```python
from build123d import *

# Parameters (mm, degrees)
SKETCH1_R           = 4
SKETCH1_R_2         = 2
BOSS_EXTRUDE1_DEPTH = 3.175


with BuildPart() as part:
    # Sketch1 → Boss-Extrude1 (new body)
    with BuildSketch(Plane.XY):
        with BuildLine():
            Line((144, -229.5), (144, -248.5))
            ThreePointArc((144, -248.5), (146.196699141, -253.803300859), (151.5, -256))
            Line((151.5, -256), (200.5, -256))
            ThreePointArc((200.5, -256), (205.803300859, -253.803300859), (208, -248.5))
            Line((208, -248.5), (208, -201.169519945))
            ThreePointArc((208, -201.169519945), (207.595148356, -198.73870325), (206.424301385, -196.570318591))
            Line((206.424301385, -196.570318591), (43.651971362, 13.099201355))
            ThreePointArc((43.651971362, 13.099201355), (41.025850524, 15.235874485), (37.727669977, 16))
            Line((37.727669977, 16), (-8.5, 16))
            ThreePointArc((-8.5, 16), (-13.803300859, 13.803300859), (-16, 8.5))
            Line((-16, 8.5), (-16, -8.5))
            ThreePointArc((-16, -8.5), (-13.803300859, -13.803300859), (-8.5, -16))
            Line((-8.5, -16), (0.5, -16))
            ThreePointArc((0.5, -16), (5.803300859, -18.196699141), (8, -23.5))
            Line((8, -23.5), (8, -214.5))
            ThreePointArc((8, -214.5), (10.196699141, -219.803300859), (15.5, -222))
            Line((15.5, -222), (136.5, -222))
            ThreePointArc((136.5, -222), (141.803300859, -224.196699141), (144, -229.5))
        make_face()
        Circle(SKETCH1_R, mode=Mode.SUBTRACT)
        with Locations((0, 8)):
            Circle(SKETCH1_R_2, mode=Mode.SUBTRACT)
        with Locations((160, -240)):
            Circle(SKETCH1_R, mode=Mode.SUBTRACT)
        with Locations((176, -240)):
            Circle(SKETCH1_R, mode=Mode.SUBTRACT)
        with Locations((160, -232)):
            Circle(SKETCH1_R_2, mode=Mode.SUBTRACT)
        with Locations((168, -240)):
            Circle(SKETCH1_R_2, mode=Mode.SUBTRACT)
        with Locations((160, -248)):
            Circle(SKETCH1_R_2, mode=Mode.SUBTRACT)
        with Locations((152, -240)):
            Circle(SKETCH1_R_2, mode=Mode.SUBTRACT)
        with Locations((200, -240)):
            Circle(SKETCH1_R_2, mode=Mode.SUBTRACT)
        with Locations((192, -248)):
            Circle(SKETCH1_R_2, mode=Mode.SUBTRACT)
        with Locations((192, -240)):
            Circle(SKETCH1_R, mode=Mode.SUBTRACT)
        with Locations((184, -240)):
            Circle(SKETCH1_R_2, mode=Mode.SUBTRACT)
        with Locations((192, -232)):
            Circle(SKETCH1_R_2, mode=Mode.SUBTRACT)
        with Locations((8, 0)):
            Circle(SKETCH1_R_2, mode=Mode.SUBTRACT)
        with Locations((0, -8)):
            Circle(SKETCH1_R_2, mode=Mode.SUBTRACT)
        with Locations((-8, 0)):
            Circle(SKETCH1_R_2, mode=Mode.SUBTRACT)
        with Locations((36, -212)):
            Circle(SKETCH1_R_2, mode=Mode.SUBTRACT)
        with Locations((28, -204)):
            Circle(SKETCH1_R_2, mode=Mode.SUBTRACT)
        with Locations((36, -196)):
            Circle(SKETCH1_R_2, mode=Mode.SUBTRACT)
        with Locations((44, -204)):
            Circle(SKETCH1_R_2, mode=Mode.SUBTRACT)
        with Locations((44, -188)):
            Circle(SKETCH1_R_2, mode=Mode.SUBTRACT)
        with Locations((36, -180)):
            Circle(SKETCH1_R_2, mode=Mode.SUBTRACT)
        with Locations((28, -188)):
            Circle(SKETCH1_R_2, mode=Mode.SUBTRACT)
        with Locations((44, -172)):
            Circle(SKETCH1_R_2, mode=Mode.SUBTRACT)
        with Locations((36, -164)):
            Circle(SKETCH1_R_2, mode=Mode.SUBTRACT)
        with Locations((28, -172)):
            Circle(SKETCH1_R_2, mode=Mode.SUBTRACT)
        with Locations((44, -156)):
            Circle(SKETCH1_R_2, mode=Mode.SUBTRACT)
        with Locations((36, -148)):
            Circle(SKETCH1_R_2, mode=Mode.SUBTRACT)
        with Locations((28, -156)):
            Circle(SKETCH1_R_2, mode=Mode.SUBTRACT)
        with Locations((44, -140)):
            Circle(SKETCH1_R_2, mode=Mode.SUBTRACT)
        with Locations((36, -132)):
            Circle(SKETCH1_R_2, mode=Mode.SUBTRACT)
        with Locations((28, -140)):
            Circle(SKETCH1_R_2, mode=Mode.SUBTRACT)
        with Locations((44, -124)):
            Circle(SKETCH1_R_2, mode=Mode.SUBTRACT)
        with Locations((36, -116)):
            Circle(SKETCH1_R_2, mode=Mode.SUBTRACT)
        with Locations((28, -124)):
            Circle(SKETCH1_R_2, mode=Mode.SUBTRACT)
        with Locations((44, -108)):
            Circle(SKETCH1_R_2, mode=Mode.SUBTRACT)
        with Locations((36, -100)):
            Circle(SKETCH1_R_2, mode=Mode.SUBTRACT)
        with Locations((28, -108)):
            Circle(SKETCH1_R_2, mode=Mode.SUBTRACT)
        with Locations((44, -92)):
            Circle(SKETCH1_R_2, mode=Mode.SUBTRACT)
        with Locations((36, -84)):
            Circle(SKETCH1_R_2, mode=Mode.SUBTRACT)
        with Locations((28, -92)):
            Circle(SKETCH1_R_2, mode=Mode.SUBTRACT)
        with Locations((44, -76)):
            Circle(SKETCH1_R_2, mode=Mode.SUBTRACT)
        with Locations((36, -68)):
            Circle(SKETCH1_R_2, mode=Mode.SUBTRACT)
        with Locations((28, -76)):
            Circle(SKETCH1_R_2, mode=Mode.SUBTRACT)
    extrude(amount=BOSS_EXTRUDE1_DEPTH)


solid = part.part
```
Build history of the part. All positions in model axes, mm. Round coordinates to 2 decimals unless told otherwise and drop trailing zeros. Loops run counter-clockwise (first coordinate to the right, second up) from the corner with the lowest first, then second, coordinate; pieces in that order, holes last. Notation, with made-up numbers: M 26.25,35.25 L 39.25,35.25 A23 ccw 39.25,48.25 Z; hole C -25,31.25 d7. An arc over 180 degrees is marked long. Answer as CSV lines item,"result".
1. Two-plate mould, pull along X, no slides. Class faces 1 (the cylindrical face through (146.139, -253.745, 1.565)), 2 (the flat face through (70, -118, 0)), 3 (the cylindrical face through (-0.867, -3.905, 1.565)): released by +X, released by -X, zero draft, split by the parting line, or undercut.
Resolved:
face 1,"released by -X"
face 2,"zero draft"
face 3,"undercut"
2. Wall check: probe 1 along Y at (x, z) = (192, 1.2); probe 2 along Y at (x, z) = (0, 1); probe 3 along X at (y, z) = (-154.5, 2.35). Give the ranges that are in metal, low to high. Write a range as [from, to].
Resolved:
probe 1,"y = [-256, -250], [-246, -244], [-236, -234], [-230, -177.99]"
probe 2,"y = [-16, -10], [-6, -4], [4, 6], [10, 16]"
probe 3,"x = [8, 26.68], [29.32, 42.68], [45.32, 173.76]"
3. Cut at B-B on x = 20.5. Write the cut outline in (y, z) (3 decimals), then the cut area to 3 significant figures.
Resolved:
outline,"M -222,0 L 16,0 L 16,3.175 L -222,3.175 Z"
area,"756 mm²"
4. Cut at A-A on z = 0.7. Count the separate pieces of the cut face and the enclosed holes in it, then the cut area to 3 significant figures.
Resolved:
separate pieces,"1"
enclosed holes,"44"
area,"31,900 mm²"
5. Cut at C-C on y = -47. Write the cut outline in (x, z) (3 decimals), then the cut area to 3 significant figures.
Resolved:
outline,"M 8,0 L 90.309,0 L 90.309,3.175 L 8,3.175 Z"
area,"261 mm²"
6. Flat gauge pins, fed straight in: P1, Ø3.5, axis at x = 28, y = -156, coming from the -Z side; P2, Ø6.5, axis at x = 36, y = -164, coming from the +Z side (3 decimals); P3, Ø1, axis at x = 148.5, z = 0.5, coming from the +Y side. Where does each tip first touch, or does it go through?
Resolved:
P1,"passes through"
P2,"stops at z = 3.175"
P3,"stops at y = -121.31"
